The drawing under review shows one solid part. Ordinate dimensions are in mm from its lowest x, y, z. A direction names the side the tool comes from. Give positions to 0.01 mm unless a question says otherwise; leave off trailing zeros. Loops run counter-clockwise (first coordinate to the right, second up) from the corner with the lowest first, then second, coordinate; pieces in that order, holes last. Notation, with made-up numbers: M -14,-17 L 41,-17 A9 ccw 41,-1 Z; hole C 79.25,-10.75 d6. An arc over 180 degrees is marked long. Write item = value, one per line. Start each with the question number.
1. We need section B-B on z = 5. Give the boundary of the cut face in (x, y).
2. For pin 1 (3 mm diameter, centred on x = 11.2, z = 8.4, fed in from -Y); pin 2 (1 mm diameter, centred on x = 9, y = 21, fed in from +Z); pin 3 (6 mm diameter, centred on x = 10, y = 10.5, fed in from +Z), all flat-tipped, find the tip position at first contact; note any pin that passes through.
3. Wall thickness on line 1 along X through (y, z) = (0.7, 8.4); line 2 along Y through (x, z) = (8.25, 4); line 3 along Y through (x, z) = (10.5, 5): over which ranges is each line inside the solid? List them lowest first. Write a range as from..to.
4. For the marked faces 4, 5, 6 and 7, list the 3-axis set-ups (+Z, -Z, +X, -X, +Y, -Y) from which the entire face can be reached by the end or side of a thin tool; tool diameter is ignored.
5. We need section A-A on x = 3.8. Give the boundary of the cut face in (y, z), then the cut area to 3 significant figures.
6. We need section C-C on z = 8.4. Give the boundary of the cut face in (x, y).
7. Draft analysis for pull direction X (two halves, no side actions). For the marked faces 1, 2 and 3, state which applies: pulls with the +X half, pulls with the -X half, needs draft (parallel to the pull), parting line crosses it, or undercut.
8. We need section D-D on y = 3.75. Give the boundary of the cut face in (x, z), then the cut area to 4 significant figures.
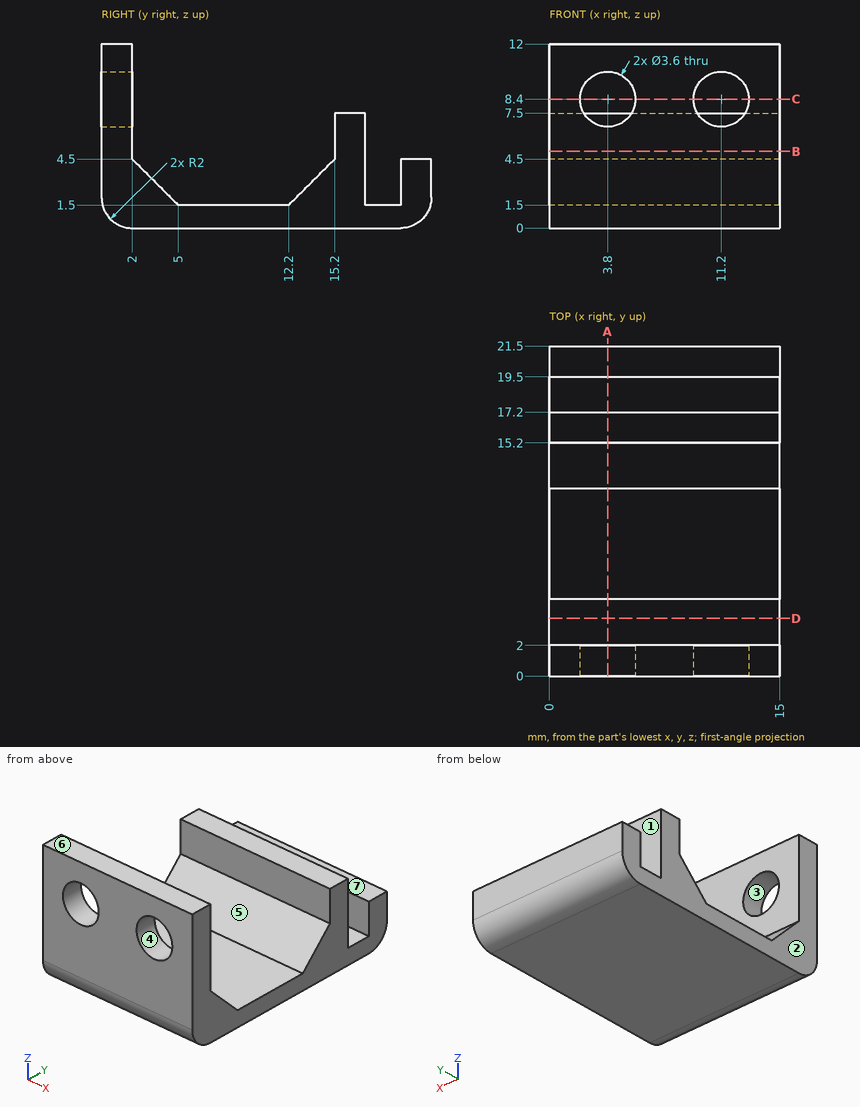
Final values:
q1.outline = M 0,0 L 15,0 L 15,2 L 0,2 Z; M 0,15.2 L 15,15.2 L 15,17.2 L 0,17.2 Z
q2.pin_1 = 15.2
q2.pin_2 = 4.5
q2.pin_3 = 2.8
q3.line_1 = 0..2, 5.6..9.4, 13..15
q3.line_2 = 0..2.5, 14.7..17.2, 19.5..21.5
q3.line_3 = 0..2, 15.2..17.2
q4.face_4 = -Y
q4.face_5 = +Z, +X, -X
q4.face_6 = +Z, +X, -X, +Y, -Y
q4.face_7 = +Z, +X, -X, +Y
q5.outline = M 0,2 A2 ccw 2,0 L 19.5,0 A2 ccw 21.5,2 L 21.5,4.5 L 19.5,4.5 L 19.5,1.5 L 17.2,1.5 L 17.2,7.5 L 15.2,7.5 L 15.2,4.5 L 12.2,1.5 L 5,1.5 L 2,4.5 L 2,6.6 L 0,6.6 Z; M 0,10.2 L 2,10.2 L 2,12 L 0,12 Z
q5.area = 71.3 mm²
q6.outline = M 0,0 L 2,0 L 2,2 L 0,2 Z; M 5.6,0 L 9.4,0 L 9.4,2 L 5.6,2 Z; M 13,0 L 15,0 L 15,2 L 13,2 Z
q7.face_1 = needs draft
q7.face_2 = pulls with the -X half
q7.face_3 = undercut
q8.outline = M 0,0 L 15,0 L 15,2.75 L 0,2.75 Z
q8.area = 41.25 mm²
